Read the model definition and answer for the solid it produces. Units are mm, in the model's axes. Face numbers are marked on the shaded views. A direction names the side the tool comes from. Round coordinates to 2 decimals unless told otherwise and drop trailing zeros. Write each loop counter-clockwise with the first axis right and the second up, starting at its lowest first coordinate (ties: lowest second). Pieces come first, ordered by that corner, then holes.
from build123d import *

# Parameters (mm, degrees)
SKETCH1_W               = 161
SKETCH1_H               = 40
BOSS_EXTRUDE1_DEPTH     = 8
SKETCH2_W               = 3
SKETCH2_H               = 40
BOSS_EXTRUDE2_DEPTH     = 20
SKETCH3_R               = 16.2
CUT_EXTRUDE1_DEPTH      = 4
SKETCH4_R               = 1.8
CUT_EXTRUDE2_DEPTH      = 1
CUT_EXTRUDE2_DEPTH_BACK = 162
CUT_EXTRUDE3_REACH      = 26
SKETCH5_R               = 13.75
FILLET1_R               = 10


with BuildPart() as part:
    # Sketch1 → Boss-Extrude1 (new body)
    with BuildSketch(Plane(origin=(0, 0, 0), x_dir=(1, 0, 0), z_dir=(0, 1, 0))):
        Rectangle(SKETCH1_W, SKETCH1_H)
    extrude(amount=BOSS_EXTRUDE1_DEPTH)

    # Sketch2 → Boss-Extrude2 (add)
    with BuildSketch(Plane(origin=(0, 8, 0), x_dir=(1, 0, 0), z_dir=(0, 1, 0))):
        with Locations((-48.5, 0)):
            Rectangle(SKETCH2_W, SKETCH2_H)
        with Locations((-79, 0)):
            Rectangle(SKETCH2_W, SKETCH2_H)
        with Locations((79, 0)):
            Rectangle(SKETCH2_W, SKETCH2_H)
        with Locations((48.5, 0)):
            Rectangle(SKETCH2_W, SKETCH2_H)
    extrude(amount=BOSS_EXTRUDE2_DEPTH)

    # Sketch3 → Cut-Extrude1 (cut)
    with BuildSketch(Plane.XZ):
        Circle(SKETCH3_R)
    extrude(amount=-CUT_EXTRUDE1_DEPTH, mode=Mode.SUBTRACT)

    # Sketch4 → Cut-Extrude2 (cut, two sides)
    with BuildSketch(Plane.ZY.offset(80.5)) as cut_extrude2_sk:
        with Locations((4, 18)):
            Circle(SKETCH4_R)
        with Locations((-4, 18)):
            Circle(SKETCH4_R)
    extrude(amount=CUT_EXTRUDE2_DEPTH, mode=Mode.SUBTRACT)
    extrude(cut_extrude2_sk.sketch, amount=-CUT_EXTRUDE2_DEPTH_BACK, mode=Mode.SUBTRACT)

    # Sketch5 → Cut-Extrude3 (cut, up to next)
    with BuildSketch(Plane.XZ.offset(-4), mode=Mode.PRIVATE) as cut_extrude3_sk1:
        Circle(SKETCH5_R)
    cut_extrude3_tool1 = extrude(cut_extrude3_sk1.sketch, amount=-CUT_EXTRUDE3_REACH, mode=Mode.PRIVATE) & part.part
    add(cut_extrude3_tool1.solids().sort_by_distance((0, 4, 0))[0], mode=Mode.SUBTRACT)

    # Fillet1
    fillet1_edges = [part.edges().sort_by_distance(p)[0] for p in [
        (-48.5, 28, 20),
        (-48.5, 28, -20),
        (-79, 28, 20),
        (-79, 28, -20),
        (79, 28, -20),
        (79, 28, 20),
        (48.5, 28, -20),
        (48.5, 28, 20),
    ]]
    fillet(fillet1_edges, radius=FILLET1_R)


solid = part.part
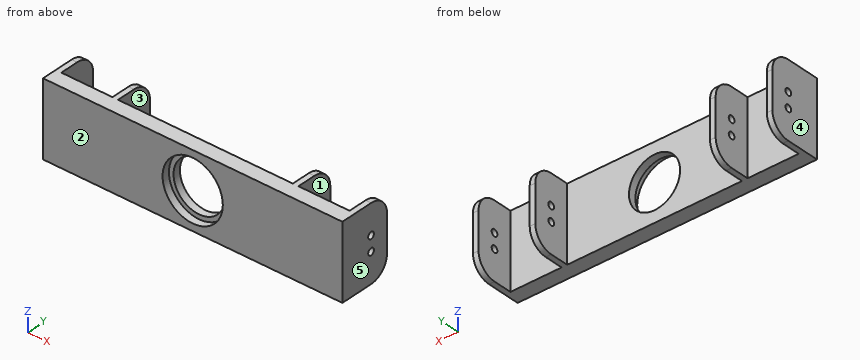
Q1. Straight lines are drawn through the part: probe 1 along X at (y, z) = (20.75, -3); probe 2 along Y at (x, z) = (49.35, -4); probe 3 along Y at (x, z) = (8.5, -15). For each, find the intervals that lie inside material, in ascending order.
Verdict:
probe 1: x = -80.5 to -77.5, -50 to -47, 47 to 50, 77.5 to 80.5
probe 2: y = 0 to 16.2, 19.8 to 28
probe 3: y = 0 to 8
Q2. Section D-D (x = 40) is taken. Determine the outline of the cut face in (y, z), then the cut area to 3 significant figures.
Verdict:
outline: (0, -20) - (8, -20) - (8, 20) - (0, 20) - close
area: 320 mm2
Q3. Which of the six approach directions +Z, -Z, +X, -X, +Y, -Y give full straight-line access (tool end or side, diameter ignored) to the marked faces 1 and 2?
Verdict:
face 1: +Z, -Z, +Y
face 2: +Z, -Z, +X, -X, -Y
Q4. Section B-B (y = 11.25) is taken. Determine the outline of the cut face in (x, z).
Verdict:
outline: (-80.5, -20) - (-77.5, -20) - (-77.5, 20) - (-80.5, 20) - close; (-50, -20) - (-47, -20) - (-47, 20) - (-50, 20) - close; (47, -20) - (50, -20) - (50, 20) - (47, 20) - close; (77.5, -20) - (80.5, -20) - (80.5, 20) - (77.5, 20) - close
Q5. Flat-ended cylindrical pins translate along their axes: pin 1 Ø5 at (x, y) = (40, 11) entering from +Z; pin 2 Ø8 at (x, z) = (-26.5, -10) entering from +Y. Find the tip coordinate at first contact, or state that the pin passes through.
Verdict:
pin 1: passes through
pin 2: stops at y = 8
Q6. Determine the mould class of the marked faces 3, 4 and 5 for opening direction X: pulls with the +X half, pulls with the -X half, needs draft (parallel to the pull), parting line crosses it, or undercut.
Verdict:
face 3: undercut
face 4: pulls with the -X half
face 5: pulls with the +X half
Q7. Section C-C (z = 4) is taken. State how many separate pieces and enclosed holes the cut face has, then the cut area to 3 significant figures.
Verdict:
separate pieces: 6
enclosed holes: 0
area: 1,250 mm2
Q8. Section A-A (x = 0) is taken. Determine the outline of the cut face in (y, z), then the cut area to 3 significant figures.
Verdict:
outline: (0, -20) - (8, -20) - (8, -13.75) - (4, -13.75) - (4, -16.2) - (0, -16.2) - close; (0, 16.2) - (4, 16.2) - (4, 13.75) - (8, 13.75) - (8, 20) - (0, 20) - close
area: 80.4 mm2
